Model file for the job. Use its own axes, mm. Face numbers are marked on the shaded views. A direction names the side the tool comes from. Round coordinates to 2 decimals unless told otherwise and drop trailing zeros. Order: outer loops, then holes, each group sorted by start corner. A loop starts at its lowest first (then second) coordinate and runs counter-clockwise, first axis right, second up. Notation, with made-up numbers: M 41.5,46.5 L 67.5,46.5 A19 ccw 67.5,65.5 Z; hole C -21.5,-7.5 d6. An arc over 180 degrees is marked long. Return JSON: item names as keys, results as strings. Group by question number.
Item 1: Probe line 1 along X through (y, z) = (4.5, -8.75); line 2 along Y through (x, z) = (-4.5, -7.25); line 3 along Y through (x, z) = (0.25, -5). List the from-to ranges inside material, lowest first.
Item 2: Slice it at A-A on y = 4. Write the cut outline in (x, z), then the cut area to 3 significant figures.
Item 3: Pin check, flat tips, straight feed: pin 1 Ø1 at (y, z) = (3.5, -10.5) entering from -X; pin 2 Ø1.7 at (x, y) = (0, 6) entering from -Z; pin 3 Ø2 at (x, y) = (0.5, 14) entering from -Z. Stop position of each tip, or through.
Item 4: Which spindle directions (+Z, -Z, +X, -X, +Y, -Y) get a long thin tool onto all of the face, cutting with end or side? Do the marked faces 1, 2 and 3. Say none if no direction does.
from build123d import *

# Parameters (mm, degrees)
BOSS_EXTRUDE1_DEPTH = 0.75
BOSS_EXTRUDE2_DEPTH = 7.5


with BuildPart() as part:
    # Sketch1 → Boss-Extrude1 (new, symmetric)
    with BuildSketch(Plane(origin=(0, 0, 0), x_dir=(0, 0, -1), z_dir=(1, 0, 0))):
        Polygon((0, 0), (14, 0), (14, 18), (0, 8), align=None)
    extrude(amount=BOSS_EXTRUDE1_DEPTH, both=True)

    # Sketch2 → Boss-Extrude2 (add, symmetric)
    with BuildSketch(Plane(origin=(0, 0, 0), x_dir=(0, 0, -1), z_dir=(1, 0, 0))):
        with BuildLine():
            ThreePointArc((-4.550304812, 10.464286171), (-5.928476621, 8.851635414), (-4.315825864, 7.473463604))
            add(Edge.make_bspline(
                [(-4.315825864, 7.473463604), (-3.583243131, 7.530897713), (-2.100585043, 7.6832237), (0.68576379, 8.118340384), (3.956902233, 8.917185571), (7.520727195, 10.282481231), (10.736128846, 12.048694485), (13.599295228, 14.193658518), (16.119096641, 16.686751031), (18.30906232, 19.477622478), (19.58868963, 21.545750976), (20.174187061, 22.599110502)],
                knots=[0, 0, 0, 0, 0.0625, 0.125, 0.25, 0.375, 0.5, 0.625, 0.75, 0.875, 1, 1, 1, 1], degree=3))
            ThreePointArc((20.174187061, 22.599110502), (19.591855999, 24.638936606), (17.552029895, 24.056605543))
            add(Edge.make_bspline(
                [(-4.550304812, 10.464286171), (6.637685906, 11.341418876), (13.172377699, 16.177239873), (17.552029895, 24.056605543)],
                knots=[0, 0, 0, 0, 1, 1, 1, 1], degree=3))
        make_face()
    extrude(amount=BOSS_EXTRUDE2_DEPTH, both=True)


solid = part.part
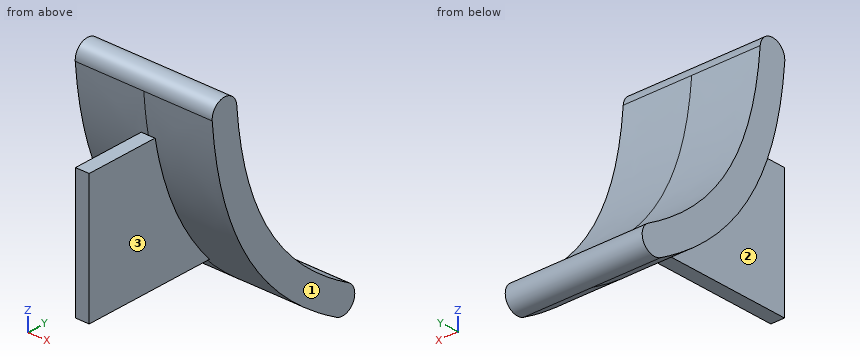
Output values:
{
 "1": {"line 1": "-0.75 to 0.75", "line 2": "10.25 to 13.59", "line 3": "0 to 12.55"},
 "2": {"outline": "M -0.75,-14 L 0.75,-14 L 0.75,0 L -0.75,0 Z", "area": "21.0 mm²"},
 "3": {"pin 1": "x = -0.75", "pin 2": "z = -14", "pin 3": "z = -14.37"},
 "4": {"face 1": "+Z, -Z, +X, +Y, -Y", "face 2": "-Z, -X, -Y", "face 3": "-Z, +X, -Y"}
}
